from build123d import *

# Parameters (mm, degrees)
F0_R     = 2
F0_W     = 19
F0_H     = 32
F0_R_2   = 2.5
F1_DEPTH = 1
F2_DEPTH = 7
F0_W_2   = 0.8
F0_H_2   = 33
F0_W_3   = 0.7
F3_DEPTH = 12.5
F4_DEPTH = 5.8
F5_R     = 1


with BuildPart() as f1:
    # F0 (on Top) → F1 (new body)
    with BuildSketch(Plane.XY):
        Polygon((85, 35), (-85, 35), (-85, 16), (-66, 16), (-66, -16), (-85, -16), (-85, -35), (85, -35), (85, -16.5), (84.3, -16.5), (84.3, 16.5), (85, 16.5), align=None)
        with Locations((-74, -24)):
            Circle(F0_R, mode=Mode.SUBTRACT)
        with Locations((74, -24)):
            Circle(F0_R, mode=Mode.SUBTRACT)
        with Locations((-74, 24)):
            Circle(F0_R, mode=Mode.SUBTRACT)
        with Locations((74, 24)):
            Circle(F0_R, mode=Mode.SUBTRACT)
        with Locations((-75.5, 0)):
            Rectangle(F0_W, F0_H)
        with Locations((-73.3, 0)):
            Circle(F0_R_2, mode=Mode.SUBTRACT)
    extrude(amount=F1_DEPTH)

    # F0 (on Top) → F2 (join)
    with BuildSketch(Plane.XY):
        with Locations((-75.5, 0)):
            Rectangle(F0_W, F0_H)
        with Locations((-73.3, 0)):
            Circle(F0_R_2, mode=Mode.SUBTRACT)
    extrude(amount=F2_DEPTH)

    # F0 (on Top) → F3 (join)
    with BuildSketch(Plane.XY):
        Polygon((-85, 16), (-85, 35), (85, 35), (85, 16.5), (85.8, 16.5), (85.8, 35.8), (-85.8, 35.8), (-85.8, -35.8), (85.8, -35.8), (85.8, -16.5), (85, -16.5), (85, -35), (-85, -35), (-85, -16), align=None)
        with Locations((85.4, 0)):
            Rectangle(F0_W_2, F0_H_2)
        with Locations((84.65, 0)):
            Rectangle(F0_W_3, F0_H_2)
    extrude(amount=F3_DEPTH)

    # F0 (on Top) → F4 (cut)
    with BuildSketch(Plane.XY):
        with Locations((85.4, 0)):
            Rectangle(F0_W_2, F0_H_2)
        with Locations((84.65, 0)):
            Rectangle(F0_W_3, F0_H_2)
    extrude(amount=F4_DEPTH, mode=Mode.SUBTRACT)

    # F5
    f5_edges = [f1.edges().sort_by_distance(p)[0] for p in [
        (-75.5, -16, 7),
        (-75.5, 16, 7),
        (-66, 0, 7),
    ]]
    fillet(f5_edges, radius=F5_R)


solid = f1.part
Check sheet for the modelled part. Datum: model origin and axes. Units: mm. A direction names the side the tool comes from. Round coordinates to 2 decimals unless told otherwise and drop trailing zeros. Loops run counter-clockwise (first coordinate to the right, second up) from the corner with the lowest first, then second, coordinate; pieces in that order, holes last. Notation, with made-up numbers: (-5, 43.25) -> (19, 43.25) arc R22 cw to (19, 63.25) -> close; hole circle Ø2 at (29.25, -21). An arc over 180 degrees is marked (long way). Put each result on its own line as item: value. Start each with the question number.
1. Draft check along Y on faces 3 (the face through (-1, 1, 0)), 4 (the face through (-1, -35.8, 6)), 5 (the face through (1, 35.8, 6)), 6 (the face through (-75.3, -1.5, 3.5)). Enter one of: +Y half, -Y half, draft (parallel to the pull), parting line (faces both ways), or undercut.
2. Section check D-D (x = 74). Enter the section's corners in (y, z).
3. Section check C-C (z = 2.5). Enter the section's corners in (x, y), plus the area to 3 significant figures.
4. Section check B-B (y = 0). Enter the section's corners in (x, z), plus the area to 3 significant figures.
5. Gauge pin test, flat ends, axial feed: pin 1 (3.5 mm diameter, centred on x = -74, y = -24, fed in from +Z); pin 2 (6 mm diameter, centred on x = -27.5, y = -24, fed in from +Z); pin 3 (2 mm diameter, centred on y = 10.5, z = 4, fed in from +X); pin 4 (8 mm diameter, centred on x = -73.3, y = 0, fed in from +Z). Record the tip position at first contact, or that the pin passes through.
6. Access from +Z, -Z, +X, -X, +Y, -Y to the whole of each face (thin tool, end or side, straight path). Record for faces 1 (the face through (-72.092, -23.399, 0.493)), 2 (the face through (-85, 0, 8)).
7. Scan lines: probe 1 along Y at (x, z) = (74, 0.45); probe 2 along X at (y, z) = (26, 8.5); probe 3 along Y at (x, z) = (52.5, 4.25). Record each from-to range of solid material in increasing order.
8. Section check A-A (x = -74). Enter the section's corners in (y, z).
Findings:
1. face 3: draft
1. face 4: -Y half
1. face 5: +Y half
1. face 6: undercut
2. outline: (-35.8, 0) -> (-26, 0) -> (-26, 1) -> (-35, 1) -> (-35, 12.5) -> (-35.8, 12.5) -> close; (-22, 0) -> (22, 0) -> (22, 1) -> (-22, 1) -> close; (26, 0) -> (35.8, 0) -> (35.8, 12.5) -> (35, 12.5) -> (35, 1) -> (26, 1) -> close
3. outline: (-85.8, -35.8) -> (85.8, -35.8) -> (85.8, -16.5) -> (85, -16.5) -> (85, -35) -> (-85, -35) -> (-85, -16) -> (-66, -16) -> (-66, 16) -> (-85, 16) -> (-85, 35) -> (85, 35) -> (85, 16.5) -> (85.8, 16.5) -> (85.8, 35.8) -> (-85.8, 35.8) -> close; hole circle Ø5 at (-73.3, 0)
3. area: 949 mm^2
4. outline: (-85.8, 0) -> (-75.8, 0) -> (-75.8, 7) -> (-85, 7) -> (-85, 12.5) -> (-85.8, 12.5) -> close; (-70.8, 0) -> (84.3, 0) -> (84.3, 1) -> (-66, 1) -> (-66, 6) arc R1 ccw to (-67, 7) -> (-70.8, 7) -> close; (84.3, 5.8) -> (85.8, 5.8) -> (85.8, 12.5) -> (84.3, 12.5) -> close
4. area: 268 mm^2
5. pin 1: passes through
5. pin 2: stops at z = 1
5. pin 3: stops at x = -66
5. pin 4: stops at z = 7
6. face 1: +Z, -Z
6. face 2: +Z
7. probe 1: y = -35.8 to -26, -22 to 22, 26 to 35.8
7. probe 2: x = -85.8 to -85, 85 to 85.8
7. probe 3: y = -35.8 to -35, 35 to 35.8
8. outline: (-35.8, 0) -> (-26, 0) -> (-26, 1) -> (-35, 1) -> (-35, 12.5) -> (-35.8, 12.5) -> close; (-22, 0) -> (-2.4, 0) -> (-2.4, 7) -> (-15, 7) arc R1 ccw to (-16, 6) -> (-16, 1) -> (-22, 1) -> close; (2.4, 0) -> (22, 0) -> (22, 1) -> (16, 1) -> (16, 6) arc R1 ccw to (15, 7) -> (2.4, 7) -> close; (26, 0) -> (35.8, 0) -> (35.8, 12.5) -> (35, 12.5) -> (35, 1) -> (26, 1) -> close
